```python
from build123d import *

# Parameters (mm, degrees)
SKETCH1_W          = 0.508
SKETCH1_H          = 0.508
SKETCH2_R          = 0.1524
CUT_EXTRUDE1_DEPTH = 12.821237499


with BuildPart() as part:
    # Sweep1: sweep along a curve in space
    with BuildLine() as sweep1_path:
        Line((0, 0, 0), (5.08, 0, 0))
        Line((5.08, 0, 0), (5.08, -10.16, 0))
        Line((5.08, -10.16, 0), (0, -10.16, 0))
        Line((0, -10.16, 0), (0, 0, 0))
    # Sketch1 → Sweep1 (sweep)
    with BuildSketch(Plane(origin=(0, 0, 0), x_dir=(0, 0, -1), z_dir=(1, 0, 0))):
        Rectangle(SKETCH1_W, SKETCH1_H)
    sweep(path=sweep1_path.line, transition=Transition.RIGHT)

    # Sketch2 → Cut-Extrude1 (cut, through all)
    with BuildSketch(Plane(origin=(5.334, 0, 0), x_dir=(0, 0, -1), z_dir=(1, 0, 0))):
        with Locations((0, -0.508)):
            Circle(SKETCH2_R)
    cut_extrude1 = extrude(amount=-CUT_EXTRUDE1_DEPTH, mode=Mode.SUBTRACT)

    # Mirror1: Cut-Extrude1 across plane
    add(cut_extrude1.mirror(Plane.ZX.offset(-5.08)), mode=Mode.SUBTRACT)


solid = part.part
```
Here's how the part is built. I have some questions about the finished solid (model axes, mm). Coordinates: 2 decimals unless noted, no trailing zeros. Order: outer loops, then holes, each group sorted by start corner. A loop starts at its lowest first (then second) coordinate and runs counter-clockwise, first axis right, second up.
1) Imagine slicing it at B-B on z = 0. List the corners of the cut face in (x, y) for me, and give its area (3 significant figures).
2) I need wall thicknesses on line 1 (Y direction, x = -0.1, z = 0); line 2 (X direction, y = -3.75, z = -0.1); line 3 (Y direction, x = 3.15, z = 0.05). Which ranges of each line are inside material? Lowest first, please.
3) Will this pin go through, and if not, where does the flat tip stop? pin 1 (2 mm diameter, centred on x = 2.5, y = -9, fed in from +Z).
4) Imagine slicing it at C-C on y = -6.25. List the corners of the cut face in (x, z) for me.
5) Imagine slicing it at A-A on x = 4.3. List the corners of the cut face in (y, z) for me.
Response values:
1. outline: (-0.25, -10.41) - (5.33, -10.41) - (5.33, -9.8) - (4.83, -9.8) - (4.83, -9.91) - (0.25, -9.91) - (0.25, -9.8) - (-0.25, -9.8) - close; (-0.25, -9.5) - (0.25, -9.5) - (0.25, -0.66) - (-0.25, -0.66) - close; (-0.25, -0.36) - (0.25, -0.36) - (0.25, -0.25) - (4.83, -0.25) - (4.83, -0.36) - (5.33, -0.36) - (5.33, 0.25) - (-0.25, 0.25) - close; (4.83, -9.5) - (5.33, -9.5) - (5.33, -0.66) - (4.83, -0.66) - close
1. area: 14.9 mm2
2. line 1: y = -10.41 to -9.8, -9.5 to -0.66, -0.36 to 0.25
2. line 2: x = -0.25 to 0.25, 4.83 to 5.33
2. line 3: y = -10.41 to -9.91, -0.25 to 0.25
3. pin 1: stops at z = 0.25
4. outline: (-0.25, -0.25) - (0.25, -0.25) - (0.25, 0.25) - (-0.25, 0.25) - close; (4.83, -0.25) - (5.33, -0.25) - (5.33, 0.25) - (4.83, 0.25) - close
5. outline: (-10.41, -0.25) - (-9.91, -0.25) - (-9.91, 0.25) - (-10.41, 0.25) - close; (-0.25, -0.25) - (0.25, -0.25) - (0.25, 0.25) - (-0.25, 0.25) - close
